Design review of the part built by this model. Coordinates are the model's own, in mm. Face numbers are marked on the shaded views. A direction names the side the tool comes from. Coordinates: 2 decimals unless noted, no trailing zeros. Write each loop counter-clockwise with the first axis right and the second up, starting at its lowest first coordinate (ties: lowest second). Pieces come first, ordered by that corner, then holes. Notation, with made-up numbers: M 52,-30.75 L 102,-30.75 A20 cw 102,6.25 Z; hole C 18.5,-3.75 d3. An arc over 180 degrees is marked long. One line per question, with ' | ' between items.
from build123d import *

# Parameters (mm, degrees)
SKETCH1_W           = 100
SKETCH1_H           = 12
BOSS_EXTRUDE1_DEPTH = 40
SKETCH3_R           = 25
SKETCH3_R_2         = 15
BOSS_EXTRUDE3_DEPTH = 20
SKETCH8_W           = 16
SKETCH8_H           = 12
CUT_EXTRUDE3_DEPTH  = 20
SKETCH9_W           = 16
SKETCH9_H           = 12
CUT_EXTRUDE4_DEPTH  = 20


with BuildPart() as part:
    # Sketch1 → Boss-Extrude1 (new body)
    with BuildSketch(Plane(origin=(0, 0, 0), x_dir=(0, 0, -1), z_dir=(1, 0, 0))):
        with Locations((15.090909091, -0.181818182)):
            Rectangle(SKETCH1_W, SKETCH1_H)
    extrude(amount=-BOSS_EXTRUDE1_DEPTH)

    # Sketch3 → Boss-Extrude3 (add, symmetric)
    with BuildSketch(Plane(origin=(0, 5.818181818, 0), x_dir=(1, 0, 0), z_dir=(0, 1, 0))):
        with Locations((-15.870623847, 15.090909091)):
            Circle(SKETCH3_R)
        with Locations((-17.470623847, 15.090909091)):
            Circle(SKETCH3_R_2, mode=Mode.SUBTRACT)
    extrude(amount=BOSS_EXTRUDE3_DEPTH, both=True)

    # Sketch8 → Cut-Extrude3 (cut)
    with BuildSketch(Plane.XY.offset(34.909090909)):
        with Locations((-20, -0.181818182)):
            Rectangle(SKETCH8_W, SKETCH8_H)
    extrude(amount=-CUT_EXTRUDE3_DEPTH, mode=Mode.SUBTRACT)

    # Sketch9 → Cut-Extrude4 (cut)
    with BuildSketch(Plane(origin=(0, 0, -65.090909091), x_dir=(-1, 0, 0), z_dir=(0, 0, -1))):
        with Locations((20, -0.181818182)):
            Rectangle(SKETCH9_W, SKETCH9_H)
    extrude(amount=-CUT_EXTRUDE4_DEPTH, mode=Mode.SUBTRACT)


solid = part.part
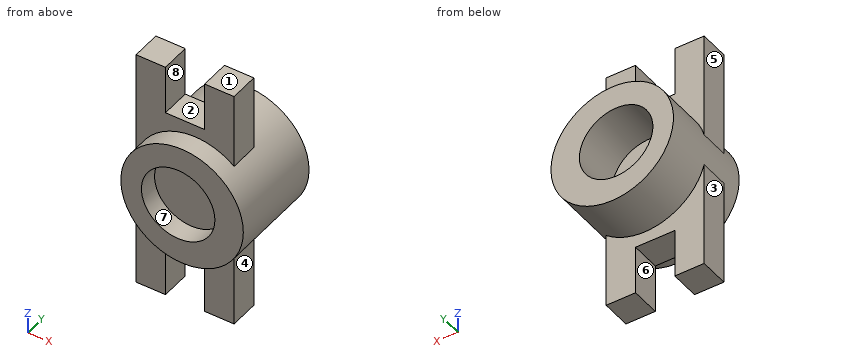
1. Take a section at A-A (z = -59). Write out the cut boundary in (x, y), then the cut area to 3 significant figures.
Answer sheet:
outline: M -40,-6.18 L -28,-6.18 L -28,5.82 L -40,5.82 Z; M -12,-6.18 L 0,-6.18 L 0,5.82 L -12,5.82 Z | area: 288 mm^2
2. Draft analysis for pull direction X (two halves, no side actions). For the marked faces 1, 2, 3 and 4, state which applies: pulls with the +X half, pulls with the -X half, needs draft (parallel to the pull), parting line crosses it, or undercut.
Answer sheet:
face 1: needs draft | face 2: undercut | face 3: pulls with the -X half | face 4: pulls with the +X half
3. Take a section at D-D (y = -8). Write out the cut boundary in (x, z).
Answer sheet:
outline: C -15.87,-15.09 d50; hole C -17.47,-15.09 d30
4. To check wall thickness, follow line 1 along X through (y, z) = (-2, -57.5); line 2 along Y through (x, z) = (-9.5, -42); line 3 along X through (y, z) = (-2, -35). State the ranges of each line that lie inside material, in increasing order. Write a range as [from, to].
Answer sheet:
line 1: [-40, -28], [-12, 0] | line 2: [-6.18, 5.82] | line 3: [-40, 0]
5. Take a section at C-C (x = -31). Write out the cut boundary in (y, z), then the cut area to 3 significant figures.
Answer sheet:
outline: M -14.18,-34.99 L -6.18,-34.99 L -6.18,-65.09 L 5.82,-65.09 L 5.82,-34.99 L 25.82,-34.99 L 25.82,-21.57 L 5.82,-21.57 L 5.82,-8.61 L 25.82,-8.61 L 25.82,4.81 L 5.82,4.81 L 5.82,34.91 L -6.18,34.91 L -6.18,4.81 L -14.18,4.81 L -14.18,-8.61 L -6.18,-8.61 L -6.18,-21.57 L -14.18,-21.57 Z | area: 1,950 mm^2
6. Insertion check: pin 1 Ø9.5 at (y, z) = (-0.5, -45) entering from -X; pin 2 Ø10 at (x, z) = (-29, -51.5) entering from +Y; pin 3 Ø13 at (y, z) = (1.5, 20.5) entering from +X. Each pin has a flat end and moves straight along its axis. Give the tip position at first contact, or say it passes through.
Answer sheet:
pin 1: x = -40 | pin 2: y = 5.82 | pin 3: x = 0
7. Take a section at B-B (y = -1). Write out the cut boundary in (x, z).
Answer sheet:
outline: M -40,-65.09 L -28,-65.09 L -28,-45.09 L -12,-45.09 L -12,-65.09 L 0,-65.09 L 0,-34.41 A25 ccw 0,4.23 L 0,34.91 L -12,34.91 L -12,14.91 L -28,14.91 L -28,34.91 L -40,34.91 L -40,-8.55 A25 ccw -40,-21.63 Z
8. Tool access review of the marked faces 5, 6, 7 and 8: name each direction out of +Z, -Z, +X, -X, +Y, -Y from which nothing blocks a thin tool from reaching the whole face with its end or side.
Answer sheet:
face 5: +Z, -X, +Y, -Y | face 6: -Z, +Y, -Y | face 7: -Y | face 8: +Z, +Y, -Y
